Verification items for this drawing (mm, ordinates from the low corner). A direction names the side the tool comes from. Round coordinates to 2 decimals unless told otherwise and drop trailing zeros. Order: outer loops, then holes, each group sorted by start corner. A loop starts at its lowest first (then second) coordinate and runs counter-clockwise, first axis right, second up. Notation, with made-up numbers: (79, 84) - (86, 84) arc R19 ccw to (86, 121) - close; hole circle Ø4 at (83.5, 6.5). An arc over 180 degrees is marked (long way). One line per question, with ' | ' between items. Start each with the question number.
Q1. Gauge pin test, flat ends, axial feed: P1, Ø0.9, axis at x = 20, y = 3, coming from the +Z side; P2, Ø1.5, axis at x = 18.5, y = 6.5, coming from the -Z side. Record the tip position at first contact, or that the pin passes through.
Q2. Tool access check on the marked faces 5 and 6. Record the directions out of +Z, -Z, +X, -X, +Y, -Y that give a thin tool (end or side, any length) a straight path to the whole face; none if there is none.
Q3. Mould release check, pull along Y, two halves, no side actions. Record for the marked faces 1, 2, 3 and 4: +Y half, -Y half, draft (parallel to the pull), parting line (faces both ways), or undercut.
Q4. Sectioned sample at A-A, the plane z = 1.75. Enter the section's corners in (x, y).
Q5. Sectioned sample at C-C, the plane y = 2.5. Enter the section's corners in (x, z), then the cut area to 3 significant figures.
Q6. Material ranges on line 1 along Y through (x, z) = (9.5, 6.35); line 2 along Y through (x, z) = (14.75, 3.5); line 3 along X through (y, z) = (18.5, 5.5), recorded low to high.
Q7. Sectioned sample at B-B, the plane x = 9.5. Enter the section's corners in (y, z).
Q8. Sectioned sample at D-D, the plane x = 5.25. Enter the section's corners in (y, z), then the cut area to 3 significant figures.
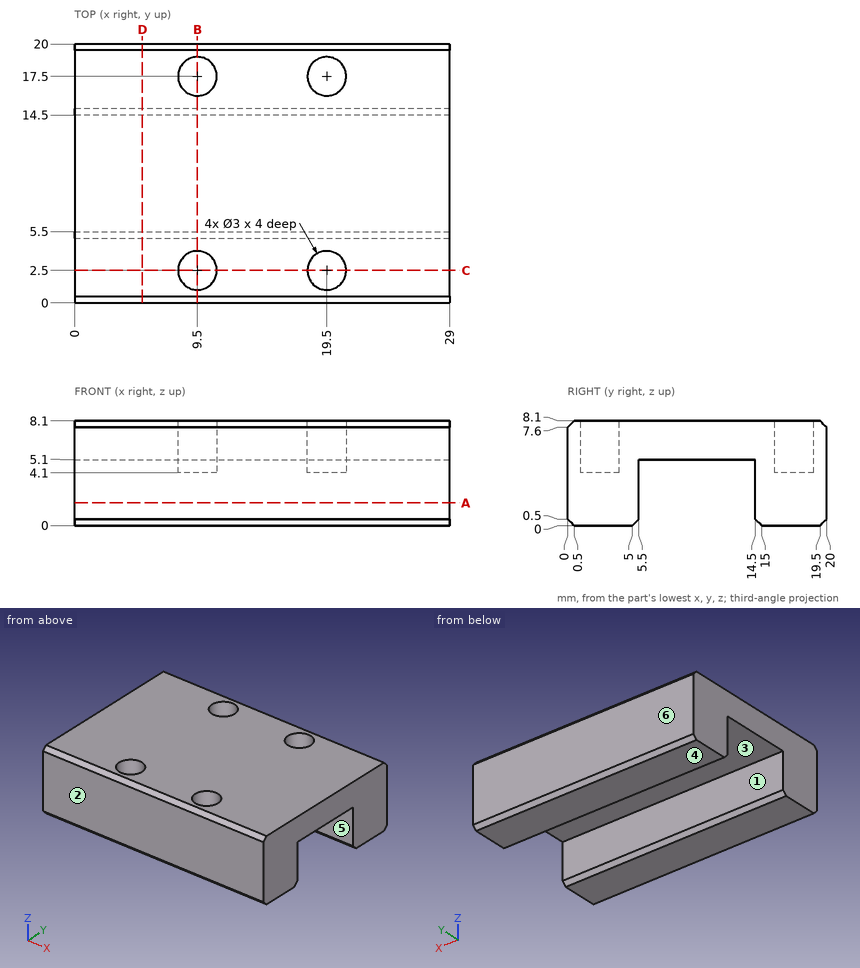
Determined:
1) P1: stops at z = 4.1 | P2: stops at z = 5.1
2) face 5: -Z, +X, -X | face 6: +Z, -Z, +X, -X, +Y
3) face 1: undercut | face 2: -Y half | face 3: undercut | face 4: draft
4) outline: (0, 0) - (29, 0) - (29, 5.5) - (0, 5.5) - close; (0, 14.5) - (29, 14.5) - (29, 20) - (0, 20) - close
5) outline: (0, 0) - (29, 0) - (29, 8.1) - (21, 8.1) - (21, 4.1) - (18, 4.1) - (18, 8.1) - (11, 8.1) - (11, 4.1) - (8, 4.1) - (8, 8.1) - (0, 8.1) - close | area: 211 mm2
6) line 1: y = 0 to 1, 4 to 16, 19 to 20 | line 2: y = 0 to 5.5, 14.5 to 20 | line 3: x = 0 to 8.38, 10.62 to 18.38, 20.62 to 29
7) outline: (0, 0.5) - (0.5, 0) - (5, 0) - (5.5, 0.5) - (5.5, 5.1) - (14.5, 5.1) - (14.5, 0.5) - (15, 0) - (19.5, 0) - (20, 0.5) - (20, 7.6) - (19.5, 8.1) - (19, 8.1) - (19, 4.1) - (16, 4.1) - (16, 8.1) - (4, 8.1) - (4, 4.1) - (1, 4.1) - (1, 8.1) - (0.5, 8.1) - (0, 7.6) - close
8) outline: (0, 0.5) - (0.5, 0) - (5, 0) - (5.5, 0.5) - (5.5, 5.1) - (14.5, 5.1) - (14.5, 0.5) - (15, 0) - (19.5, 0) - (20, 0.5) - (20, 7.6) - (19.5, 8.1) - (0.5, 8.1) - (0, 7.6) - close | area: 115 mm2
